from build123d import *

# Parameters (mm, degrees)
BOSS_EXTRUDE1_DEPTH = 25
SHELL1_T            = -3
SKETCH2_R           = 15
BOSS_EXTRUDE2_DEPTH = 70
SKETCH3_R           = 12
CUT_EXTRUDE1_DEPTH  = 75
SKETCH4_R           = 15
BOSS_EXTRUDE3_DEPTH = 70
SKETCH5_R           = 12
CUT_EXTRUDE2_DEPTH  = 75


with BuildPart() as part:
    # Sketch1 → Boss-Extrude1 (new body, symmetric)
    with BuildSketch(Plane.XY):
        with BuildLine():
            Line((0, 71.51248035), (0, 121.51248035))
            ThreePointArc((0, 121.51248035), (86.020520014, 85.518075871), (123.192898424, 0))
            Line((123.192898424, 0), (73.192898424, 0))
            ThreePointArc((73.192898424, 0), (50.686723581, 50.177611321), (0, 71.51248035))
        make_face()
    extrude(amount=BOSS_EXTRUDE1_DEPTH, both=True)

    # Shell1
    shell1_openings = [part.faces().sort_by_distance(p)[0] for p in [
        (58.725035505, 58.052041885, 25),
    ]]
    offset(amount=SHELL1_T, openings=shell1_openings, kind=Kind.INTERSECTION)

    # Sketch2 → Boss-Extrude2 (add)
    with BuildSketch(Plane.ZY):
        with Locations((0, 96.51248035)):
            Circle(SKETCH2_R)
    extrude(amount=BOSS_EXTRUDE2_DEPTH)

    # Sketch3 → Cut-Extrude1 (cut)
    with BuildSketch(Plane.ZY.offset(70)):
        with Locations((0, 96.51248035)):
            Circle(SKETCH3_R)
    extrude(amount=-CUT_EXTRUDE1_DEPTH, mode=Mode.SUBTRACT)

    # Sketch4 → Boss-Extrude3 (add)
    with BuildSketch(Plane.XZ):
        with Locations((98.192898424, 0)):
            Circle(SKETCH4_R)
    extrude(amount=BOSS_EXTRUDE3_DEPTH)

    # Sketch5 → Cut-Extrude2 (cut)
    with BuildSketch(Plane.XZ.offset(70)):
        with Locations((98.192898424, 0)):
            Circle(SKETCH5_R)
    extrude(amount=-CUT_EXTRUDE2_DEPTH, mode=Mode.SUBTRACT)


solid = part.part
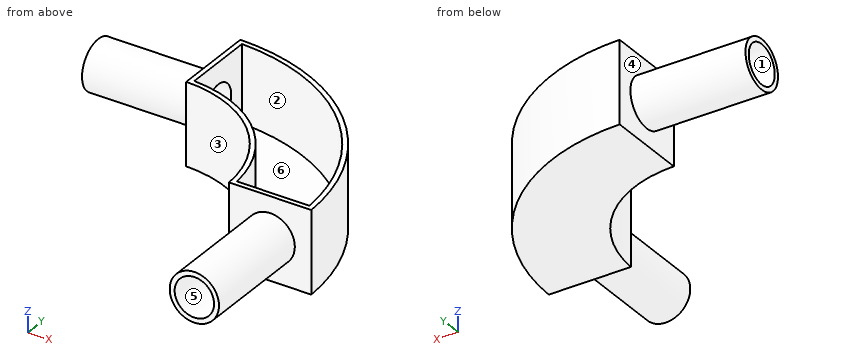
Input: part model. Units: mm. Frame: model coordinates. Face numbers are marked on the shaded views. A direction names the side the tool comes from. Give positions to 0.01 mm unless a question says otherwise; leave off trailing zeros. Order: outer loops, then holes, each group sorted by start corner. A loop starts at its lowest first (then second) coordinate and runs counter-clockwise, first axis right, second up. Notation, with made-up numbers: (13.25, 47.25) - (67.25, 47.25) arc R17 ccw to (67.25, 76.25) - close; hole circle Ø10 at (75.25, 11). An arc over 180 degrees is marked (long way). Answer as a JSON object with one key per item and string values. Group by question number.
Q1. Cut plane B-B, the plane x = 102.5. Output: boundary loops of the cut face in (y, z).
Q2. Cut plane D-D, the plane x = 22.5. Output: boundary loops of the cut face in (y, z), then the cut area to 3 significant figures.
Q3. Set-up query: the marked faces 4, 5 and 6. Return all of +Z, -Z, +X, -X, +Y, -Y with unobstructed straight access to the full face (end or side cutting, diameter ignored); none if empty.
Q4. Cut plane C-C, the plane z = 17.5. Output: boundary loops of the cut face in (x, y).
Q5. Mould query, pull axis X, two halves, no side actions, for the marked faces 1, 2 and 3. Classes: pulls with the +X half, pulls with the -X half, needs draft (parallel to the pull), parting line crosses it, or undercut.
Q6. Cut plane A-A, the plane z = 0. Output: boundary loops of the cut face in (x, y).
Q7. Line query: probe 1 along Y at (x, z) = (-42, 0); probe 2 along Y at (x, z) = (104, 17); probe 3 along X at (y, z) = (42, 16.5). Output: solid intervals per line, ascending.
Q8. First-contact query: pin 1 Ø10 at (x, z) = (68.5, -11) entering from -Y; pin 2 Ø1.5 at (y, z) = (9, -2.5) entering from +X; pin 3 Ø4 at (x, z) = (7, 7) entering from -Y. Flat tips, straight axial feed; report the tip coordinate or a pass-through.
Results:
{
 "1": {"outline": "(-70, -14.37) - (0, -14.37) - (0, -25) - (65.48, -25) - (65.48, 25) - (59.88, 25) - (59.88, -22) - (3, -22) - (3, -11.2) - (-70, -11.2) - close; (-70, 11.2) - (3, 11.2) - (3, 25) - (0, 25) - (0, 14.37) - (-70, 14.37) - close"},
 "2": {"outline": "(67.51, -25) - (119.15, -25) - (119.15, 25) - (116.09, 25) - (116.09, -22) - (70.67, -22) - (70.67, 25) - (67.51, 25) - close", "area": "447 mm^2"},
 "3": {"face 4": "-X", "face 5": "-Y", "face 6": "+Z"},
 "4": {"outline": "(0, 71.51) arc R75 cw to (73.19, 0) - (123.19, 0) arc R125 ccw to (0, 121.51) - close; hole (3, 74.39) arc R78 cw to (76, 3) - (120.07, 3) arc R122 ccw to (3, 118.43) - close"},
 "5": {"face 1": "needs draft", "face 2": "undercut", "face 3": "pulls with the -X half"},
 "6": {"outline": "(-70, 81.51) - (0, 81.51) - (0, 71.51) arc R75 cw to (73.19, 0) - (83.19, 0) - (83.19, -70) - (86.19, -70) - (86.19, 3) - (76, 3) arc R78 ccw to (3, 74.39) - (3, 84.51) - (-70, 84.51) - close; (-70, 108.51) - (3, 108.51) - (3, 118.43) arc R122 cw to (120.07, 3) - (110.19, 3) - (110.19, -70) - (113.19, -70) - (113.19, 0) - (123.19, 0) arc R125 ccw to (0, 121.51) - (0, 111.51) - (-70, 111.51) - close"},
 "7": {"probe 1": "81.51 to 84.51, 108.51 to 111.51", "probe 2": "0 to 3, 57.34 to 63.16", "probe 3": "57.92 to 61.65, 111.45 to 114.68"},
 "8": {"pin 1": "y = 0", "pin 2": "x = 122.69", "pin 3": "y = 70.76"}
}
